from build123d import *

# Parameters (mm, degrees)
BOSS_EXTRUDE1_DEPTH = 45
RIB1_REACH          = 86.595
SKETCH3_WALL_W      = 202.812019758
SKETCH3_WALL_H      = 6
SKETCH5_R           = 6
CUT_EXTRUDE1_DEPTH  = 90
SKETCH6_R           = 6
CUT_EXTRUDE2_DEPTH  = 90
SKETCH7_R           = 10
BOSS_EXTRUDE2_DEPTH = 37.5
RIB2_REACH          = 112.482
SKETCH8_WALL_W      = 290.231918176
SKETCH8_WALL_H      = 6


with BuildPart() as part:
    # Sketch1 → Boss-Extrude1 (new, symmetric)
    with BuildSketch(Plane.XY):
        Polygon((0, 0), (27.5, 0), (27.5, -10), (67.5, -10), (67.5, 0), (37.5, 0), (37.5, 10), (-37.5, 10), (-37.5, 0), (-67.5, 0), (-67.5, -10), (-27.5, -10), (-27.5, 0), align=None)
    extrude(amount=BOSS_EXTRUDE1_DEPTH, both=True)

    # Sketch3 wall → Rib1 (add, up to next)
    with BuildSketch(Plane(origin=(52.5, 5, 5), x_dir=(0.948683298051, -0.316227766017, 0), z_dir=(0.316227766017, 0.948683298051, 0)), mode=Mode.PRIVATE) as rib1_sk1:
        Rectangle(SKETCH3_WALL_W, SKETCH3_WALL_H)
    rib1_tool1 = extrude(rib1_sk1.sketch, amount=-RIB1_REACH, mode=Mode.PRIVATE) - part.part
    rib1 = rib1_tool1.solids().sort_by_distance((52.5, 5, 5))[0]
    add(rib1)

    # Mirror1: Rib1 across plane
    add(rib1.mirror(Plane(origin=(0, 0, 0), x_dir=(0, 0, 1), z_dir=(1, 0, 0))))

    # Sketch5 → Cut-Extrude1 (cut)
    with BuildSketch(Plane(origin=(0, 0, 0), x_dir=(1, 0, 0), z_dir=(0, 1, 0))):
        with Locations(Location((53, -25, 0), (0, 0, 180))):
            Circle(SKETCH5_R)
    cut_extrude1 = extrude(amount=-CUT_EXTRUDE1_DEPTH, mode=Mode.SUBTRACT)

    # Mirror2: Cut-Extrude1 across plane
    add(cut_extrude1.mirror(Plane(origin=(0, 0, 0), x_dir=(0, 0, 1), z_dir=(1, 0, 0))), mode=Mode.SUBTRACT)

    # Sketch6 → Cut-Extrude2 (cut)
    with BuildSketch(Plane(origin=(0, 0, 0), x_dir=(1, 0, 0), z_dir=(0, 1, 0))):
        with Locations(Location((53, 25, 0), (0, 0, 180))):
            Circle(SKETCH6_R)
    cut_extrude2 = extrude(amount=-CUT_EXTRUDE2_DEPTH, mode=Mode.SUBTRACT)

    # Mirror3: Cut-Extrude2 across plane
    add(cut_extrude2.mirror(Plane(origin=(0, 0, 0), x_dir=(0, 0, 1), z_dir=(1, 0, 0))), mode=Mode.SUBTRACT)

    # Sketch7 → Boss-Extrude2 (add, symmetric)
    with BuildSketch(Plane(origin=(0, 0, 0), x_dir=(0, 0, -1), z_dir=(1, 0, 0))):
        with BuildLine():
            Line((5, 10), (45, 10))
            Line((45, 10), (45, 55))
            ThreePointArc((45, 55), (25, 75), (5, 55))
            Line((5, 55), (5, 10))
        make_face()
        with Locations((25, 55)):
            Circle(SKETCH7_R, mode=Mode.SUBTRACT)
    extrude(amount=BOSS_EXTRUDE2_DEPTH, both=True)

    # Sketch8 wall → Rib2 (add, up to next)
    with BuildSketch(Plane(origin=(0, 32.5, 20), x_dir=(0, -0.668964731622, 0.743294146247), z_dir=(0, -0.743294146247, -0.668964731622)), mode=Mode.PRIVATE) as rib2_sk1:
        Rectangle(SKETCH8_WALL_W, SKETCH8_WALL_H)
    rib2_tool1 = extrude(rib2_sk1.sketch, amount=RIB2_REACH, mode=Mode.PRIVATE) - part.part
    add(rib2_tool1.solids().sort_by_distance((0, 32.5, 20))[0])


solid = part.part
Model file for the job. Use its own axes, mm. A direction names the side the tool comes from. Give positions to 0.01 mm unless a question says otherwise; leave off trailing zeros. Loops run counter-clockwise (first coordinate to the right, second up) from the corner with the lowest first, then second, coordinate; pieces in that order, holes last. Notation, with made-up numbers: (0.5, -37) -> (25.5, -37) arc R24 cw to (25.5, -27) -> close; hole circle Ø3 at (51, -32.75). An arc over 180 degrees is marked (long way). Use a Markdown table: item, result. Add a question column.
(1) Slice it at D-D on x = -18.5. List the corners of the cut face in (y, z).
(2) Wall check: line 1 along Z through (x, y) = (-53, -6); line 2 along X through (y, z) = (41, -25.5); line 3 along Y through (x, z) = (25.5, -28). Give the ranges that are in metal, low to high.
(3) Slice it at B-B on z = 25. List the corners of the cut face in (x, y).
(4) Slice it at A-A on z = -25. List the corners of the cut face in (x, y).
(5) Drop flat-ended pins along their axis: pin 1 Ø15 at (x, z) = (-49.5, -26.5) entering from +Y; pin 2 Ø17 at (x, z) = (-27.5, 15.5) entering from +Y; pin 3 Ø12 at (x, y) = (10.5, 34) entering from +Z; pin 4 Ø12 at (y, z) = (55, -25) entering from +X. Give the stop position or say it passes through.
(6) Mould opens along X. For faces 5 (the flat face through (-52.29, 5.07, 4.96)), 6 (the cylindrical face through (-59, -5, 25)), 7 (the flat face through (-48, -10, 1)) say: +X half, -X half, draft (parallel to the pull), parting line (faces both ways), or undercut.
(7) Slice it at C-C on x = 53. List the corners of the cut face in (y, z), and give its area (3 significant figures).
(8) Tool access for faces 1 (the flat face through (-3, 23, 11)), 2 (the flat face through (0, 0, 1)), 3 (the flat face through (48, 4, 8)), 4 (the flat face through (-48, 4, 2)): list every direction of +Z, -Z, +X, -X, +Y, -Y with a clear straight run to the whole face (end or side of a thin tool).
Filled sheet:
| question | item | result |
|---|---|---|
| 1 | outline | (0, -45) -> (55, -45) arc R20 ccw to (55, -5) -> (10, -5) -> (10, 45) -> (0, 45) -> close; hole circle Ø20 at (55, -25) |
| 2 | line 1 | -45 to -31, -19 to 19, 31 to 45 |
| 2 | line 2 | -37.5 to 37.5 |
| 2 | line 3 | 0 to 45.46, 64.54 to 74.77 |
| 3 | outline | (-67.5, -10) -> (-59, -10) -> (-59, 0) -> (-67.5, 0) -> close; (-47, -10) -> (-27.5, -10) -> (-27.5, 0) -> (27.5, 0) -> (27.5, -10) -> (47, -10) -> (47, 0) -> (37.5, 0) -> (37.5, 10) -> (3, 10) -> (3, 28) -> (-3, 28) -> (-3, 10) -> (-37.5, 10) -> (-37.5, 0) -> (-47, 0) -> close; (59, -10) -> (67.5, -10) -> (67.5, 0) -> (59, 0) -> close |
| 4 | outline | (-67.5, -10) -> (-59, -10) -> (-59, 0) -> (-67.5, 0) -> close; (-47, -10) -> (-27.5, -10) -> (-27.5, 0) -> (27.5, 0) -> (27.5, -10) -> (47, -10) -> (47, 0) -> (37.5, 0) -> (37.5, 45) -> (-37.5, 45) -> (-37.5, 0) -> (-47, 0) -> close; (-37.5, 65) -> (37.5, 65) -> (37.5, 75) -> (-37.5, 75) -> close; (59, -10) -> (67.5, -10) -> (67.5, 0) -> (59, 0) -> close |
| 5 | pin 1 | y = 0 |
| 5 | pin 2 | y = 10 |
| 5 | pin 3 | z = -5 |
| 5 | pin 4 | through |
| 6 | face 5 | -X half |
| 6 | face 6 | undercut |
| 6 | face 7 | draft |
| 7 | outline | (-10, -45) -> (0, -45) -> (0, -31) -> (-10, -31) -> close; (-10, -19) -> (0, -19) -> (0, 2) -> (4.83, 2) -> (4.83, 8) -> (0, 8) -> (0, 19) -> (-10, 19) -> close; (-10, 31) -> (0, 31) -> (0, 45) -> (-10, 45) -> close |
| 7 | area | 689 mm2 |
| 8 | face 1 | +Z, -X, +Y |
| 8 | face 2 | +Z, -Z, -Y |
| 8 | face 3 | +Z, +X, +Y |
| 8 | face 4 | -Z, -X, +Y |
